Verification items for the finished model (mm, model axes). Round coordinates to 2 decimals unless told otherwise and drop trailing zeros. Write each loop counter-clockwise with the first axis right and the second up, starting at its lowest first coordinate (ties: lowest second). Pieces come first, ordered by that corner, then holes. Notation, with made-up numbers: (69, 57) - (120, 57) arc R24 cw to (120, 92) - close; hole circle Ø10 at (-11.5, 20). An arc over 180 degrees is marked (long way). Answer as a JSON object with one key per item and string values.
```python
from build123d import *

# Parameters (mm, degrees)
REDONDEO3_R           = 3
CROQUIS9_R            = 3
CORTAR_EXTRUIR3_DEPTH = 18


with BuildPart() as part:
    # Croquis4 → Revolución4 (revolve)
    with BuildSketch(Plane.XY):
        with BuildLine():
            Line((20, -17.912835745), (20, 22.083900585))
            Line((20, 22.083900585), (18, 22.083900585))
            Line((18, 22.083900585), (18, 25.087164255))
            Line((18, 25.087164255), (20, 25.087164255))
            ThreePointArc((20, 25.087164255), (14.142135624, 39.229299878), (0, 45.087164255))
            Line((0, 45.087164255), (0, -17.912835745))
            Line((0, -17.912835745), (20, -17.912835745))
        make_face()
    revolve(axis=Axis((0, 45.087164255, 0), (0, -1, 0)))

    # Redondeo3
    redondeo3_edges = [part.edges().sort_by_distance(p)[0] for p in [
        (-20, -17.912835745, 0),
    ]]
    fillet(redondeo3_edges, radius=REDONDEO3_R)

    # Croquis9 → Cortar-Extruir3 (cut)
    with BuildSketch(Plane(origin=(0, 0, 0), x_dir=(0, 0, -1), z_dir=(1, 0, 0))):
        with Locations((8, 33.885616094)):
            Circle(CROQUIS9_R)
        with Locations((-8, 33.885616094)):
            Circle(CROQUIS9_R)
    extrude(amount=CORTAR_EXTRUIR3_DEPTH, mode=Mode.SUBTRACT)


solid = part.part
```
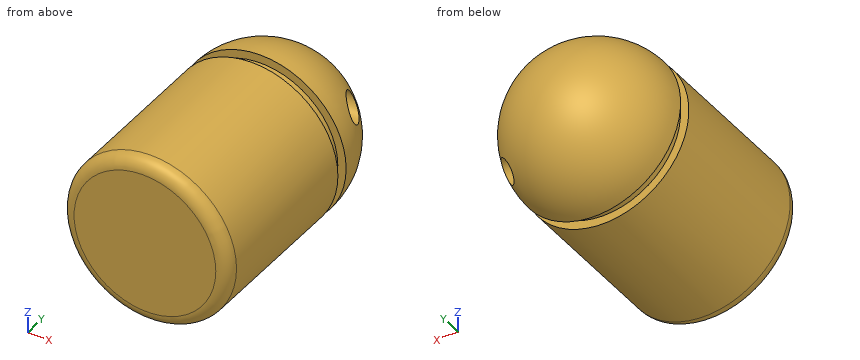
Q1. Material ranges on line 1 along Z through (x, y) = (6, 33); line 2 along Y through (x, z) = (6, 8); line 3 along Z through (x, y) = (13.5, 33.5), recorded low to high. Write a range as [from, to].
Geometry check:
{"line 1": "z = [-17.36, -10.87], [-5.13, 5.13], [10.87, 17.36]", "line 2": "y = [-17.91, 30.89], [36.89, 42.41]", "line 3": "z = [-12.12, -10.98], [-5.02, 5.02], [10.98, 12.12]"}
Q2. Section check C-C, the plane x = 3. State how many separate pieces and enclosed holes the cut face has, then the cut area to 3 significant figures.
Geometry check:
{"separate pieces": "1", "enclosed holes": "2", "area": "2,240 mm2"}
Q3. Gauge pin test, flat ends, axial feed: P1, Ø5, axis at y = 33.89, z = 8, coming from the -X side; P2, Ø4, axis at y = 12, z = -9, coming from the +X side (3 decimals); P3, Ø1, axis at y = 20.5, z = -14, coming from the +X side. Record the tip position at first contact, or that the pin passes through.
Geometry check:
{"P1": "stops at x = -17.66", "P2": "stops at x = 18.735", "P3": "stops at x = 14.76"}
Q4. Section check B-B, the plane y = 0. Record the cut outline in (x, z), then the cut area to 3 significant figures.
Geometry check:
{"outline": "circle Ø40 at (0, 0)", "area": "1,260 mm2"}
Q5. Section check A-A, the plane z = 0. Record the cut outline in (x, y).
Geometry check:
{"outline": "(-20, -14.91) arc R3 ccw to (-17, -17.91) - (17, -17.91) arc R3 ccw to (20, -14.91) - (20, 22.08) - (18, 22.08) - (18, 25.09) - (20, 25.09) arc R20 ccw to (-20, 25.09) - (-18, 25.09) - (-18, 22.08) - (-20, 22.08) - close"}
